Source: CAD feature listing. Evaluate the final solid. Frame: model axes, mm. Round coordinates to 2 decimals unless told otherwise and drop trailing zeros. Order: outer loops, then holes, each group sorted by start corner. A loop starts at its lowest first (then second) coordinate and runs counter-clockwise, first axis right, second up. Notation, with made-up numbers: (-32, 25) -> (3, 25) arc R13 cw to (3, 38) -> close; hole circle Ø6 at (37, 60.25). An arc over 180 degrees is marked (long way). Answer as CSV lines item,"result".
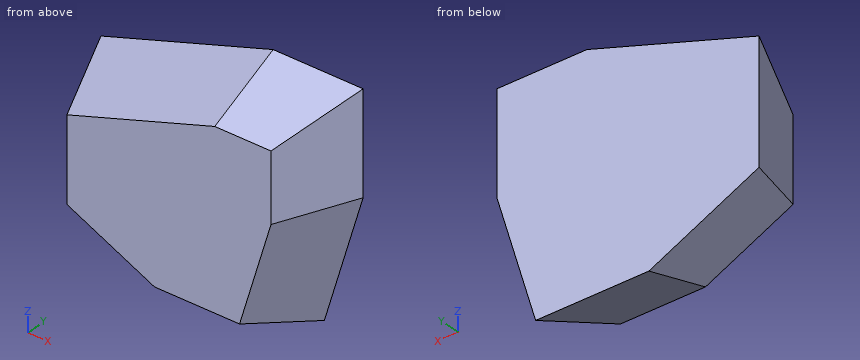
from build123d import *

# Parameters (mm, degrees)
EXTRUDE_1_DEPTH = 25
DRAFT_1_ANGLE   = 20


with BuildPart() as part:
    # 草图1 → 凸台-拉伸1 (new body)
    with BuildSketch(Plane(origin=(0, 0, 0), x_dir=(1, 0, 0), z_dir=(0, 1, 0))):
        Polygon((-61.640527642, 14.993641859), (-61.640527642, -11.384061411), (-15.271301893, -26.933023339), (2.359472358, -26.933023339), (2.359472358, -5.275540654), (-7.496820929, 28.066976661), (-34.152184234, 28.066976661), align=None)
    extrude(amount=EXTRUDE_1_DEPTH)

    # 拔模1
    draft_1_faces = [part.faces().sort_by_distance(p)[0] for p in [
        (-38.455914768, 12.5, 19.158542375),
        (-61.640527642, 12.5, -1.804790224),
        (-47.896355938, 12.5, -21.53030926),
        (-20.824502582, 12.5, -28.066976661),
        (-2.568674286, 12.5, -11.395718003),
        (2.359472358, 12.5, 16.104281997),
        (-6.455914768, 12.5, 26.933023339),
    ]]
    draft(draft_1_faces, Plane(origin=(0, 0, 0), x_dir=(0, 0, -1), z_dir=(0, -1, 0)), DRAFT_1_ANGLE)


solid = part.part
1. Section query C-C on x = -2.5. Return loops of the section in (y, z).
Results below:
outline,"(0, -11.16) -> (18.37, -34.75) -> (25, -37.17) -> (25, 36.03) -> (0, 26.93) -> close"
2. Line query: L1, parallel to Z at x = -8, y = 12; L2, parallel to X at y = 3, z = -4; L3, parallel to X at y = 6, z = 5.5. Output: solid intervals per line, ascending. Write a range as [from, to].
Results below:
L1,"[-32.43, 31.3]"
L2,"[-62.73, 0.76]"
L3,"[-63.82, 4.54]"
3. Section query D-D on y = 23.25. Return loops of the section in (x, z).
Results below:
outline,"(-70.1, -20.34) -> (-36.06, -36.53) -> (-1.17, -36.53) -> (10.82, 4.05) -> (10.82, 35.4) -> (-16.65, 35.4) -> (-70.1, 17.47) -> close"
4. Section query A-A on y = 8.25. Return loops of the section in (x, z), and give its area (3 significant figures).
Results below:
outline,"(-64.64, -16.89) -> (-34.83, -31.07) -> (-5.25, -31.07) -> (5.36, 4.84) -> (5.36, 29.94) -> (-15.76, 29.94) -> (-64.64, 13.54) -> close"
area,"3,470 mm2"
5. Section query B-B on z = -19.5. Return loops of the section in (x, y).
Results below:
outline,"(-70.74, 25) -> (-68.77, 19.6) -> (-52.17, 0) -> (-4.96, 0) -> (4.52, 25) -> close"
6. Pin query (flat end, axial travel): pin 1 (12 mm diameter, centred on x = -40, y = 10, fed in from +Z); pin 2 (5 mm diameter, centred on x = -33, y = 18, fed in from -Z); pin 3 (4 mm diameter, centred on y = 3.5, z = -20, fed in from -X). Return the tip coordinate at first contact, or that it passes through.
Results below:
pin 1,"z = 25.54"
pin 2,"z = -35.53"
pin 3,"x = -58.61"
